The model under review builds one solid part; all positions refer to its coordinate system, in mm. Face numbers are marked on the shaded views. A direction names the side the tool comes from. Give positions to 0.01 mm unless a question says otherwise; leave off trailing zeros. Loops run counter-clockwise (first coordinate to the right, second up) from the corner with the lowest first, then second, coordinate; pieces in that order, holes last. Notation, with made-up numbers: (82.25, -1) - (89.25, -1) arc R22 ccw to (89.25, 31) - close; hole circle Ø9 at (34.5, 31.5). An arc over 180 degrees is marked (long way). Return JSON: item names as keys, results as strings. Group by question number.
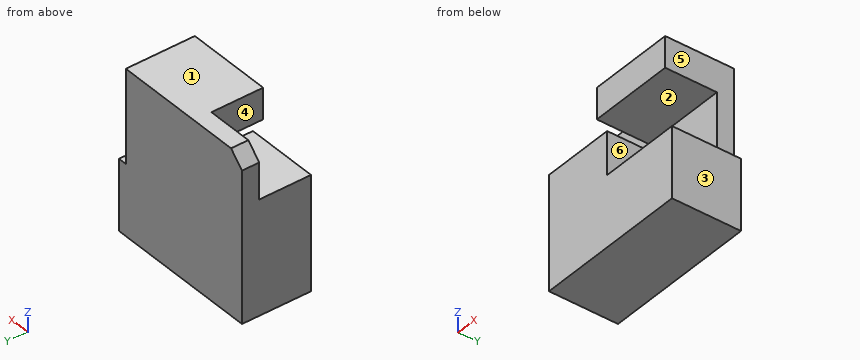
from build123d import *

# Parameters (mm, degrees)
PAD_DEPTH       = 20
SKETCH001_W     = 2.5
SKETCH001_H     = 27
POCKET_DEPTH    = 20.001
POCKET001_DEPTH = 15


with BuildPart() as part:
    # Sketch → Pad (new body)
    with BuildSketch(Plane.XZ):
        Polygon((23.748329, 0), (-21.251671, 0), (-21.251671, 43.5), (-17.251671, 47.5), (23.748329, 47.5), align=None)
    extrude(amount=PAD_DEPTH)

    # Sketch001 → Pocket (cut, through all)
    with BuildSketch(Plane.XZ.offset(20)):
        with Locations((22.498329, 34)):
            Rectangle(SKETCH001_W, SKETCH001_H)
    extrude(amount=-POCKET_DEPTH, mode=Mode.SUBTRACT)

    # Sketch002 → Pocket001 (cut)
    with BuildSketch(Plane.XZ.offset(20)):
        Polygon((21.248329, 20.5), (0, 20.5), (0, 33), (-21.251671, 33), (-21.251671, 47.5), (-3.751671, 47.5), (-3.751671, 38.5), (21.248329, 38.5), align=None)
    extrude(amount=-POCKET001_DEPTH, mode=Mode.SUBTRACT)


solid = part.part
Item 1: Take a section at B-B (x = -3). State the section outline as (y, z) points.
Item 2: Take a section at A-A (y = -16.5). State the section outline as (x, z) points, then the cut area to 3 significant figures.
Item 3: Take a section at C-C (y = -3.75). State the section outline as (x, z) points, then the cut area to 3 significant figures.
Item 4: For P1, Ø4, axis at y = -12.5, z = 24, coming from the +X side; P2, Ø7, axis at y = -11.5, z = 41, coming from the -X side, all flat-tipped, find the tip position at first contact; note any pin that passes through.
Item 5: Take a section at D-D (z = 37.5). State the section outline as (x, y) points, then the cut area to 4 significant figures.
Item 6: Mouldability with a two-part tool opening along Z and no side actions: class the marked faces 1, 2 and 3 as +Z half, -Z half, draft (parallel to the pull), parting line (faces both ways), or undercut.
Item 7: Tool access review of the marked faces 4, 5 and 6: name each direction out of +Z, -Z, +X, -X, +Y, -Y from which nothing blocks a thin tool from reaching the whole face with its end or side.
Item 8: For L1, parallel to Z at x = 6, y = -17.5; L2, parallel to X at y = -2.75, z = 30.5; L3, parallel to Y at x = 14, z = 25.5, list the stretches that pass through material, from the lowest coordinate up. Write a range as from..to.
Check sheet entries:
{
 "1": {"outline": "(-20, 0) - (0, 0) - (0, 47.5) - (-20, 47.5) - (-20, 38.5) - (-5, 38.5) - (-5, 33) - (-20, 33) - close"},
 "2": {"outline": "(-21.25, 0) - (23.75, 0) - (23.75, 20.5) - (0, 20.5) - (0, 33) - (-21.25, 33) - close; (-3.75, 38.5) - (21.25, 38.5) - (21.25, 47.5) - (-3.75, 47.5) - close", "area": "1,410 mm^2"},
 "3": {"outline": "(-21.25, 0) - (23.75, 0) - (23.75, 20.5) - (21.25, 20.5) - (21.25, 47.5) - (-17.25, 47.5) - (-21.25, 43.5) - close", "area": "2,060 mm^2"},
 "4": {"P1": "stops at x = 0", "P2": "stops at x = -3.75"},
 "5": {"outline": "(-21.25, -5) - (21.25, -5) - (21.25, 0) - (-21.25, 0) - close", "area": "212.5 mm^2"},
 "6": {"face 1": "+Z half", "face 2": "undercut", "face 3": "draft"},
 "7": {"face 4": "+Z, -X, -Y", "face 5": "+Z, +X, +Y, -Y", "face 6": "+X, -Y"},
 "8": {"L1": "z = 0..20.5, 38.5..47.5", "L2": "x = -21.25..21.25", "L3": "y = -5..0"}
}
